Autodesk Inventor part; units mm, degrees
ref_plane "Plan YZ" through (0, 0, 0) normal (1, 0, 0) x (0, 1, 0)
ref_plane "Plan XZ" through (0, 0, 0) normal (0, 1, 0) x (-1, 0, 0)
ref_plane "Plan XY" through (0, 0, 0) normal (0, 0, 1) x (1, 0, 0)
sketch "Esquisse6" plane through (0, 0, 0) normal (0, 1, 0) x (-1, 0, 0)
  line L0 (0, 0) -> (2.548, 0)
  line L1 (2.548, 0.05) -> (1.9686, 0.6294)
  line L2 (1.5, 1.7607) -> (1.5, 7.5)
  line L3 (1, 8) -> (0, 8)
  line L4 (0, -1.6) -> (0, 9.6) construction
  line L5 (2.548, 0) -> (2.548, 0.05)
  arc A0 (1.5, 1.7607) -> (1.9686, 0.6294) centre (3.1, 1.7607) ccw
  line L6 (1.5, 7.5) -> (1, 8)
  line L7 (0, 0.6997) -> (1.4, 0.6997)
  line L8 (1.4, 0.6997) -> (0, 1.508)
  line L9 (0, 8) -> (0, 1.508)
  line L10 (0, 0.6997) -> (0, 0)
  point P0 (1.5, 8)
  dimension "d9" = 5.096
  dimension "d10" = 45
  dimension "d11" = 0.05
  dimension "d12" = 1.6
  dimension "d13" = 8
  dimension "d14" = 3
  dimension "d16" = 0.5
  dimension "d17" = 0.5
  dimension "d36" = 60
  dimension "d37" = 1.508
  dimension "d38" = 2.8
revolve "Révolution1" add sketch "Esquisse6" angle 360 about axis through (0, 0, 0) along (0, 0, 1)
sketch "Esquisse1" plane through (0, 0, 0) normal (0, 0, 1) x (1, 0, 0)
  circle A0 centre (0, 0) radius 1.15 construction
  line L0 (1.299, 2.25) -> (0, 0) construction
  line L1 (0, 3.0788) -> (0, -2.723) construction
  circle A1 centre (0, 1.15) radius 0.25 construction
  circle A2 centre (0.7761, 1.3442) radius 0.55 construction
  circle A3 centre (-0.9959, 0.575) radius 0.25 construction
  circle A4 centre (-0.7761, 1.3442) radius 0.55 construction
  circle A5 centre (-0.9959, -0.575) radius 0.25 construction
  circle A6 centre (-1.5521, 0) radius 0.55 construction
  circle A7 centre (0, -1.15) radius 0.25 construction
  circle A8 centre (-0.7761, -1.3442) radius 0.55 construction
  circle A9 centre (0.9959, -0.575) radius 0.25 construction
  circle A10 centre (0.7761, -1.3442) radius 0.55 construction
  circle A11 centre (0.9959, 0.575) radius 0.25 construction
  circle A12 centre (1.5521, 0) radius 0.55 construction
  arc A13 (0.2425, 1.2107) -> (-0.2425, 1.2107) centre (0, 1.15) ccw
  arc A14 (-0.9272, 0.8154) -> (-0.2425, 1.2107) centre (-0.7761, 1.3442) ccw
  arc A15 (-0.9272, 0.8154) -> (-1.1697, 0.3953) centre (-0.9959, 0.575) ccw
  arc A16 (-1.1697, -0.3953) -> (-1.1697, 0.3953) centre (-1.5521, 0) ccw
  arc A17 (-1.1697, -0.3953) -> (-0.9272, -0.8154) centre (-0.9959, -0.575) ccw
  arc A18 (-0.2425, -1.2107) -> (-0.9272, -0.8154) centre (-0.7761, -1.3442) ccw
  arc A19 (-0.2425, -1.2107) -> (0.2425, -1.2107) centre (0, -1.15) ccw
  arc A20 (0.9272, -0.8154) -> (0.2425, -1.2107) centre (0.7761, -1.3442) ccw
  arc A21 (0.9272, -0.8154) -> (1.1697, -0.3953) centre (0.9959, -0.575) ccw
  arc A22 (1.1697, 0.3953) -> (1.1697, -0.3953) centre (1.5521, 0) ccw
  arc A23 (1.1697, 0.3953) -> (0.9272, 0.8154) centre (0.9959, 0.575) ccw
  arc A24 (0.2425, 1.2107) -> (0.9272, 0.8154) centre (0.7761, 1.3442) ccw
  circle A25 centre (0, 0) radius 1.4 construction
  dimension "d4" = 2.3
  dimension "d2" = 30
  dimension "d18" = 0.5
  dimension "d19" = 1.1
  dimension "d25" = 360
  dimension "d39" = 2.8
extrude "Extrusion2" cut sketch "Esquisse1" along normal up to next
thread "Filetage1"
equation "\"d38\" = d39"
properties part number "ISO14581_M3x8" material "Acier zingué, clair"
Source: CAD feature listing. Evaluate the final solid. Frame: model axes, mm. Round coordinates to 2 decimals unless told otherwise and drop trailing zeros. Loops run counter-clockwise (first coordinate to the right, second up) from the corner with the lowest first, then second, coordinate; pieces in that order, holes last. Notation, with made-up numbers: M 12,47 L 37,47 A25 cw 37,65 Z; hole C -14.5,15 d8. An arc over 180 degrees is marked long. Use a Markdown table: item, result. Add a question column.
1. Ray query, line 1 along Y through (x, z) = (0, 6.25); line 2 along X through (y, z) = (-1.25, 2.75); line 3 along Y through (x, z) = (0.95, 1.5). Return the intervals inside material, ascending. Write a range as [from, to].
2. Pull-direction query (X, two-part tool) for faces 1 (the conical face through (0.18, 0.16, 1.37)), 2 (the flat face through (-1, 1, 0)), 3 (the cylindrical face through (1.5, -0.07, 4.67)); classes: +X half, -X half, draft (parallel to the pull), parting line (faces both ways), or undercut.
3. Contact query for flat-ended pins moving along their axis: pin 1 (3 mm diameter, centred on y = 1, z = 2.5, fed in from -X); pin 2 (1 mm diameter, centred on x = 1, y = -1, fed in from +Z). Output: stop coordinate, or through.
4. Cut plane A-A, the plane z = 5.75. Output: boundary loops of the cut face in (x, y), and give its area (3 significant figures).
Solution:
| question | item | result |
|---|---|---|
| 1 | line 1 | y = [-1.5, 1.5] |
| 1 | line 2 | x = [-0.83, 0.83] |
| 1 | line 3 | y = [-1.19, 1.19] |
| 2 | face 1 | undercut |
| 2 | face 2 | draft |
| 2 | face 3 | parting line |
| 3 | pin 1 | stops at x = -1.58 |
| 3 | pin 2 | stops at z = 8 |
| 4 | outline | C 0,0 d3 |
| 4 | area | 7.07 mm2 |
